Source: CAD feature listing. Evaluate the final solid. Frame: model axes, mm. A direction names the side the tool comes from. Give positions to 0.01 mm unless a question says otherwise; leave off trailing zeros. Write each loop counter-clockwise with the first axis right and the second up, starting at its lowest first coordinate (ties: lowest second). Pieces come first, ordered by that corner, then holes. Notation, with made-up numbers: M 45.25,49 L 55.25,49 A29 ccw 55.25,87 Z; hole C -30,22 d4. An arc over 180 degrees is marked long. Use CSV: the item, a comma, the result in double quotes. Start each with the question number.
from build123d import *

# Parameters (mm, degrees)
PAD001_DEPTH         = 53.3
PAD002_DEPTH         = 53.3
POCKET_DEPTH         = 18
POCKET001_DEPTH      = 5
SKETCH_W             = 0.8
SKETCH_H             = 19.4
PAD_DEPTH            = 53.3
POCKET004_DEPTH      = 19.401
POCKET004_DEPTH_BACK = -2.101
FILLET_R             = 1
FILLET001_R          = 1


with BuildPart() as part:
    # Sketch001 → Pad001 (new body, symmetric)
    with BuildSketch(Plane.XZ):
        Polygon((64.35, 0), (55.65, 0), (55.65, -19.4), (0, -19.4), (0, -16.9), (53.3, -16.9), (53.3, 2.1), (64.35, 2.1), align=None)
    pad001 = extrude(amount=PAD001_DEPTH, both=True)

    # Sketch002 → Pad002 (join, symmetric)
    with BuildSketch(Plane.XZ):
        with BuildLine():
            ThreePointArc((53, 2.1), (52.25, 1.35), (53, 0.6))
            Line((53.3, 0.6), (53, 0.6))
            Line((53.3, 2.1), (53.3, 0.6))
            Line((53.3, 2.1), (53, 2.1))
        make_face()
    pad002 = extrude(amount=PAD002_DEPTH, both=True)

    # Sketch003 → Pocket (cut)
    with BuildSketch(Plane.XY):
        with BuildLine():
            ThreePointArc((28.8, 38.3), (40.3, 26.8), (51.8, 38.3))
            Line((51.8, 38.3), (51.8, 49.3))
            ThreePointArc((51.8, 49.3), (51.214214, 50.714214), (49.8, 51.3))
            Line((30.8, 51.3), (49.8, 51.3))
            ThreePointArc((30.8, 51.3), (29.385786, 50.714214), (28.8, 49.3))
            Line((28.8, 38.3), (28.8, 49.3))
        make_face()
        with BuildLine():
            ThreePointArc((51.8, -38.3), (40.3, -26.8), (28.8, -38.3))
            Line((28.8, -38.3), (28.8, -49.3))
            ThreePointArc((28.8, -49.3), (29.385786, -50.714214), (30.8, -51.3))
            Line((30.8, -51.3), (49.8, -51.3))
            ThreePointArc((49.8, -51.3), (51.214214, -50.714214), (51.8, -49.3))
            Line((51.8, -38.3), (51.8, -49.3))
        make_face()
    pocket = extrude(amount=-POCKET_DEPTH, mode=Mode.SUBTRACT)

    # Sketch004 → Pocket001 (cut)
    with BuildSketch(Plane.XY):
        with BuildLine():
            ThreePointArc((59.8, -45.8), (60.053187, -46.603007), (60.721172, -47.11557))
            Line((60.721172, -47.11557), (64.5, -48.490951))
            Line((64.5, -42.959049), (64.5, -48.490951))
            Line((60.721172, -44.33443), (64.5, -42.959049))
            ThreePointArc((60.721172, -44.33443), (60.053187, -44.846993), (59.8, -45.65))
            Line((59.8, -45.65), (59.8, -45.8))
        make_face()
        with BuildLine():
            ThreePointArc((60.721172, 47.11557), (60.053187, 46.603007), (59.8, 45.8))
            Line((59.8, 45.8), (59.8, 45.65))
            ThreePointArc((59.8, 45.65), (60.053187, 44.846993), (60.721172, 44.33443))
            Line((60.721172, 44.33443), (64.5, 42.959049))
            Line((64.5, 48.490951), (64.5, 42.959049))
            Line((60.721172, 47.11557), (64.5, 48.490951))
        make_face()
    pocket001 = extrude(amount=POCKET001_DEPTH, mode=Mode.SUBTRACT)

    # Mirrored: Pad001, Pad002, Pocket, Pocket001 across YZ
    add(pad001.mirror(Plane.YZ))
    add(pad002.mirror(Plane.YZ))
    add(pocket.mirror(Plane.YZ), mode=Mode.SUBTRACT)
    add(pocket001.mirror(Plane.YZ), mode=Mode.SUBTRACT)

    # Sketch → Pad (join, symmetric)
    with BuildSketch(Plane.XZ):
        with Locations((56.05, -9.7)):
            Rectangle(SKETCH_W, SKETCH_H)
    extrude(amount=PAD_DEPTH, both=True)

    # Sketch005 → Pocket004 (cut, two sides)
    with BuildSketch(Plane.XY) as pocket004_sk:
        Polygon((47.3, -7.856773), (47.3, 7.856773), (53.3, 7.856773), (55.65, 6.5), (55.65, -6.5), (53.3, -7.856773), align=None)
    extrude(amount=-POCKET004_DEPTH, mode=Mode.SUBTRACT)
    extrude(pocket004_sk.sketch, amount=-POCKET004_DEPTH_BACK, mode=Mode.SUBTRACT)

    # Fillet
    fillet_edges = [part.edges().sort_by_distance(p)[0] for p in [
        (64.35, -53.3, 1.05),
        (64.35, -43.013645, 1.05),
        (64.35, -48.436355, 1.05),
        (64.35, 43.013645, 1.05),
        (64.35, 48.436355, 1.05),
        (64.35, 53.3, 1.05),
        (-64.35, 53.3, 1.05),
        (-64.35, 48.436355, 1.05),
        (-64.35, 43.013645, 1.05),
        (-64.35, -48.436355, 1.05),
        (-64.35, -53.3, 1.05),
        (-64.35, -43.013645, 1.05),
    ]]
    fillet(fillet_edges, radius=FILLET_R)

    # Fillet001
    fillet001_edges = [part.edges().sort_by_distance(p)[0] for p in [
        (55.65, -6.5, -8.65),
        (55.65, 6.5, -8.65),
        (47.3, -7.856773, -18.15),
        (47.3, 7.856773, -18.15),
    ]]
    fillet(fillet001_edges, radius=FILLET001_R)


solid = part.part
Item 1: Section B-B (z = -1.5). Return the cut outline in (x, y).
Item 2: Material intervals for probe 1 along X at (y, z) = (-29, -2.5); probe 2 along X at (y, z) = (-21, 0.5); probe 3 along Y at (x, z) = (30.5, -17), sorted ascending.
Item 3: Pull-direction query (X, two-part tool) for faces 1 (the flat face through (-55.65, -1, -10)), 2 (the flat face through (13.8, 53.3, -17.4)), 3 (the cylindrical face through (-40.553, -26.803, -17.442)), 4 (the cylindrical face through (40.553, -26.803, -17.442)); classes: released by +X, released by -X, zero draft, split by the parting line, or undercut.
Item 4: Section A-A (y = 1.5). Return the cut outline in (x, z), plus the area to 3 significant figures.
Item 5: Section C-C (x = 40.3). Return the cut outline in (y, z).
Item 6: Section D-D (y = -13.5). Return the cut outline in (x, z), plus the area to 3 significant figures.
Item 7: Set-up query: faces 5 (the flat face through (56.45, -1, -10)), 6 (the flat face through (53.3, 30, -8)), 7 (the flat face through (-40, -39, -18)). Return all of +Z, -Z, +X, -X, +Y, -Y with unobstructed straight access to the full face (end or side cutting, diameter ignored); none if empty.
Item 8: Contact query for flat-ended pins moving along their axis: pin 1 Ø3 at (y, z) = (14, -9) entering from -X; pin 2 Ø4 at (x, y) = (10, 34) entering from +Z; pin 3 Ø1 at (y, z) = (1, -11.5) entering from +X. Output: stop coordinate, or through.
Output values:
1,outline,"M -55.65,-53.3 L -53.3,-53.3 L -53.3,53.3 L -55.65,53.3 Z; M 53.3,-53.3 L 56.45,-53.3 L 56.45,53.3 L 53.3,53.3 L 53.3,7.86 L 55.15,6.79 A1 cw 55.65,5.92 L 55.65,-5.92 A1 cw 55.15,-6.79 L 53.3,-7.86 Z"
2,probe 1,"x = -55.65 to -53.3, 53.3 to 56.45"
2,probe 2,"x = -64.35 to -53.3, 53.3 to 64.35"
2,probe 3,"y = -53.3 to -51.28, -32.28 to 32.28, 51.28 to 53.3"
3,face 1,"released by -X"
3,face 2,"zero draft"
3,face 3,"undercut"
3,face 4,"undercut"
4,outline,"M -64.35,0 L -55.65,0 L -55.65,-19.4 L 47.3,-19.4 L 47.3,-16.9 L -53.3,-16.9 L -53.3,0.6 L -53,0.6 A0.75 ccw -53,2.1 L -64.35,2.1 Z; M 55.65,-19.4 L 56.45,-19.4 L 56.45,0 L 64.35,0 L 64.35,2.1 L 55.65,2.1 Z"
4,area,"355 mm2"
5,outline,"M -53.3,-19.4 L 53.3,-19.4 L 53.3,-16.9 L 51.3,-16.9 L 51.3,-18 L 26.8,-18 L 26.8,-16.9 L -26.8,-16.9 L -26.8,-18 L -51.3,-18 L -51.3,-16.9 L -53.3,-16.9 Z"
6,outline,"M -64.35,0 L -55.65,0 L -55.65,-19.4 L 56.45,-19.4 L 56.45,0 L 64.35,0 L 64.35,2.1 L 53,2.1 A0.75 ccw 53,0.6 L 53.3,0.6 L 53.3,-16.9 L -53.3,-16.9 L -53.3,0.6 L -53,0.6 A0.75 ccw -53,2.1 L -64.35,2.1 Z"
6,area,"422 mm2"
7,face 5,"-Z, +X, +Y, -Y"
7,face 6,"+Y, -Y"
7,face 7,"+Z"
8,pin 1,"stops at x = -55.65"
8,pin 2,"stops at z = -16.9"
8,pin 3,"stops at x = 56.45"
